The listing builds one solid part. Answer for the finished solid, in the listing's coordinates (mm). A direction names the side the tool comes from. Round coordinates to 2 decimals unless told otherwise and drop trailing zeros. Write each loop counter-clockwise with the first axis right and the second up, starting at its lowest first coordinate (ties: lowest second). Pieces come first, ordered by that corner, then holes.
(1) A cutting plane is placed at C-C, the plane x = -28. Give the vertices of the cut face in (y, z).
(2) Each of these flat-tipped pins is pushed along its axis until it touches: pin 1 Ø4 at (x, z) = (-28.75, 10) entering from -Y; pin 2 Ø10 at (y, z) = (76, -9) entering from -X; pin 3 Ø4 at (x, y) = (-25, 49) entering from +Z; pin 4 Ø4 at (x, y) = (-26, 66.5) entering from +Z. Where does it stop, or does it pass through?
(3) Find the intervals of material crossed by probe 1 along Z at (x, y) = (-27.75, 67.25); probe 2 along Z at (x, y) = (-28.75, 54); probe 3 along Z at (x, y) = (-29.75, 39.5), in increasing order.
(4) A cutting plane is placed at D-D, the plane y = 52.5. Give the vertices of the cut face in (x, z), and give its area (3 significant figures).
(5) A cutting plane is placed at A-A, the plane y = 67.25. Give the vertices of the cut face in (x, z), and give its area (3 significant figures).
(6) A cutting plane is placed at B-B, the plane z = 0. Give the vertices of the cut face in (x, y), and give its area (3 significant figures).
(7) The mould has two halves that part along Z. Classify faces 1 (the face through (-31.96, 56.58, -13.574)), 2 (the face through (-27, 27, 0)), 3 (the face through (-31.5, 57, 0)), 4 (the face through (-26.29, 56.58, 13.15)): +Z half, -Z half, draft (parallel to the pull), parting line (faces both ways), or undercut.
(8) For faces 5 (the face through (-32.98, 56.58, 8)), 6 (the face through (-30.25, 56.58, -9.93)), determine the directions among +Z, -Z, +X, -X, +Y, -Y from which every point of the face is accessible in a straight line to the end or side of a thin tool.
from build123d import *

# Parameters (mm, degrees)
SKETCH135_R  = 1.5
PAD107_DEPTH = 50
SKETCH138_R  = 1.5
PAD111_DEPTH = 50
SKETCH098_R  = 1.5
PAD075_DEPTH = 60


with BuildPart() as screwcutout:
    # Sketch135 → Pad107 (new body, symmetric)
    with BuildSketch(Plane(origin=(0, 34, 0), x_dir=(0, 1, 0), z_dir=(1, 0, 0))):
        with Locations((3.25, 0)):
            Circle(SKETCH135_R)
    extrude(amount=PAD107_DEPTH, both=True)


with BuildPart() as sidecutouts:
    # Sketch138 → Pad111 (new body, symmetric)
    with BuildSketch(Plane(origin=(0, 70, 0), x_dir=(0, 1, 0), z_dir=(1, 0, 0))):
        with Locations((-2.75, 0)):
            Circle(SKETCH138_R)
    extrude(amount=PAD111_DEPTH, both=True)

    # Fusion004020008: union ScrewCutout
    add(screwcutout.part)


with BuildPart() as sidewall:
    # Sketch098 → Pad075 (new body)
    with BuildSketch(Plane.XZ.offset(-27)):
        Polygon((-31.5, -4), (-31.5, 4), (-34.5, 12.107695), (-29.490381, 15), (-23, 11.252777), (-23, -11.252777), (-29.490381, -15), (-34.5, -12.107695), align=None)
        with Locations((-28.75, 10)):
            Circle(SKETCH098_R, mode=Mode.SUBTRACT)
        with Locations((-28.75, -10)):
            Circle(SKETCH098_R, mode=Mode.SUBTRACT)
    extrude(amount=-PAD075_DEPTH)

    # Cut007019013: cut sideCutouts
    add(sidecutouts.part, mode=Mode.SUBTRACT)


solid = sidewall.part
Solutions:
1. outline: (27, -14.14) - (87, -14.14) - (87, -11.3) - (27, -11.3) - close; (27, -8.7) - (87, -8.7) - (87, 8.7) - (27, 8.7) - close; (27, 11.3) - (87, 11.3) - (87, 14.14) - (27, 14.14) - close; hole circle Ø3 at (37.25, 0); hole circle Ø3 at (67.25, 0)
2. pin 1: stops at y = 27
2. pin 2: stops at x = -34.5
2. pin 3: stops at z = 13.56
2. pin 4: stops at z = 14.14
3. probe 1: z = -14 to -11.12, -8.88 to -1.5, 1.5 to 8.88, 11.12 to 14
3. probe 2: z = -14.57 to -11.5, -8.5 to 8.5, 11.5 to 14.57
3. probe 3: z = -14.85 to -11.12, -8.88 to 8.88, 11.12 to 14.85
4. outline: (-34.5, -12.11) - (-29.49, -15) - (-23, -11.25) - (-23, 11.25) - (-29.49, 15) - (-34.5, 12.11) - (-31.5, 4) - (-31.5, -4) - close; hole circle Ø3 at (-28.75, -10); hole circle Ø3 at (-28.75, 10)
4. area: 244 mm2
5. outline: (-34.5, -12.11) - (-29.49, -15) - (-23, -11.25) - (-23, -1.5) - (-31.5, -1.5) - (-31.5, -4) - close; (-34.5, 12.11) - (-31.5, 4) - (-31.5, 1.5) - (-23, 1.5) - (-23, 11.25) - (-29.49, 15) - close; hole circle Ø3 at (-28.75, -10); hole circle Ø3 at (-28.75, 10)
5. area: 218 mm2
6. outline: (-31.5, 27) - (-23, 27) - (-23, 35.75) - (-31.5, 35.75) - close; (-31.5, 38.75) - (-23, 38.75) - (-23, 65.75) - (-31.5, 65.75) - close; (-31.5, 68.75) - (-23, 68.75) - (-23, 87) - (-31.5, 87) - close
6. area: 459 mm2
7. face 1: -Z half
7. face 2: draft
7. face 3: undercut
7. face 4: +Z half
8. face 5: -X, +Y, -Y
8. face 6: +Y, -Y
